Build history of the part. All positions in model axes, mm. Face numbers are marked on the shaded views. A direction names the side the tool comes from. Give positions to 0.01 mm unless a question says otherwise; leave off trailing zeros. Order: outer loops, then holes, each group sorted by start corner. A loop starts at its lowest first (then second) coordinate and runs counter-clockwise, first axis right, second up. Notation, with made-up numbers: (-14, 11.25) - (35, 11.25) arc R15 cw to (35, 20.25) - close; hole circle Ø8 at (1, 8). An arc over 180 degrees is marked (long way). One line per item, written item: value.
```python
from build123d import *

# Parameters (mm, degrees)
F0_W     = 50.3428
F0_H     = 26.7335
F1_DEPTH = 1.6764
F2_W     = 50.3174
F2_H     = 19.1008
F3_DEPTH = 7.8867
F4_W     = 23.241
F4_H     = 17.78
F5_DEPTH = 2.794
F6_R     = 0.635
F7_DEPTH = 25.4
F8_SIZE  = 1.27


with BuildPart() as f1:
    # F0 (on Top) → F1 (new body)
    with BuildSketch(Plane.XY):
        Rectangle(F0_W, F0_H)
    extrude(amount=-F1_DEPTH)

    # F2 (on Top) → F3 (join)
    with BuildSketch(Plane.XY):
        Rectangle(F2_W, F2_H)
    extrude(amount=F3_DEPTH)

    # F4 (on face) → F5 (join)
    with BuildSketch(Plane(origin=(0, 0, -1.6764), x_dir=(1, 0, 0), z_dir=(0, 0, -1))):
        Rectangle(F4_W, F4_H)
    extrude(amount=F5_DEPTH)

    # F6 (on Top) → F7 (cut)
    with BuildSketch(Plane.XY):
        with Locations((-3.81, 11.46175)):
            Circle(F6_R)
        with Locations((-1.27, 11.46175)):
            Circle(F6_R)
        with Locations((1.27, 11.46175)):
            Circle(F6_R)
        with Locations((3.81, 11.46175)):
            Circle(F6_R)
    extrude(amount=-F7_DEPTH, mode=Mode.SUBTRACT)

    # F8
    f8_edges = [f1.edges().sort_by_distance(p)[0] for p in [
        (25.1714, 13.36675, -0.8382),
        (25.1714, -13.36675, -0.8382),
        (-25.1714, -13.36675, -0.8382),
        (-25.1714, 13.36675, -0.8382),
    ]]
    chamfer(f8_edges, length=F8_SIZE)


solid = f1.part
```
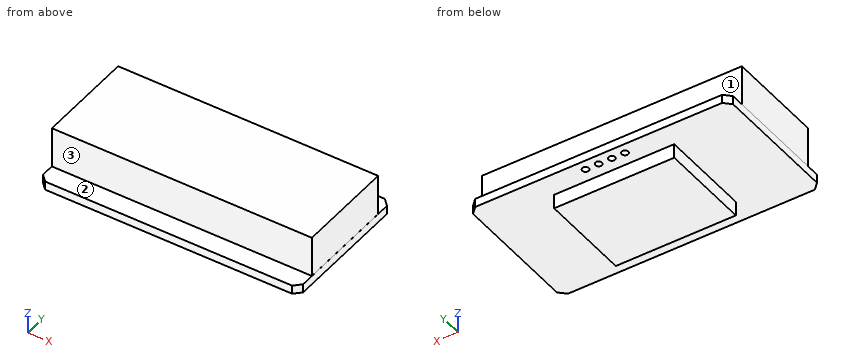
(1) Slice it at A-A, the plane x = -3.81. Give the cut face in (y, z), and give its area (3 significant figures).
Completed:
outline: (-13.37, -1.68) - (-8.89, -1.68) - (-8.89, -4.47) - (8.89, -4.47) - (8.89, -1.68) - (10.83, -1.68) - (10.83, 0) - (9.55, 0) - (9.55, 7.89) - (-9.55, 7.89) - (-9.55, 0) - (-13.37, 0) - close; (12.1, -1.68) - (13.37, -1.68) - (13.37, 0) - (12.1, 0) - close
area: 243 mm²
(2) Pin check, flat tips, straight feed: P1, Ø2, axis at y = 1.5, z = -3, coming from the -X side; P2, Ø6, axis at y = -6.5, z = 5.5, coming from the +X side; P3, Ø4, axis at y = 2.5, z = 4.5, coming from the -X side; P4, Ø6, axis at x = 13, y = -9, coming from the -Z side. Stop position of each tip, or through.
Completed:
P1: x = -11.62
P2: x = 25.16
P3: x = -25.16
P4: z = -4.47
(3) Slice it at C-C, the plane x = 15. Give the cut face in (y, z), and give its area (3 significant figures).
Completed:
outline: (-13.37, -1.68) - (13.37, -1.68) - (13.37, 0) - (9.55, 0) - (9.55, 7.89) - (-9.55, 7.89) - (-9.55, 0) - (-13.37, 0) - close
area: 195 mm²
(4) Slice it at D-D, the plane z = 4. Give the cut face in (x, y).
Completed:
outline: (-25.16, -9.55) - (25.16, -9.55) - (25.16, 9.55) - (-25.16, 9.55) - close
(5) Drill centre lines: line 1 (Y direction, x = -1.27, z = -1.15); line 2 (X direction, y = 8.75, z = 0); line 3 (Y direction, x = -17, z = 2.75). Where is each one in solid material? Low to high.
Completed:
line 1: -13.37 to 10.83, 12.1 to 13.37
line 2: -25.16 to 25.16
line 3: -9.55 to 9.55
(6) 3-axis set-ups, long thin cutter, end or side, ignore diameter. For the marked faces 1, 2 and 3: which of +Z, -Z, +X, -X, +Y, -Y reach the whole face in a straight line?
Completed:
face 1: +Z, +X, -X, +Y
face 2: +Z, +X, -X
face 3: +Z, +X, -X, -Y
